For this review, take the finished solid that the model builds, in its own axes (mm). A direction names the side the tool comes from. Round coordinates to 2 decimals unless told otherwise and drop trailing zeros. Write each loop counter-clockwise with the first axis right and the second up, starting at its lowest first coordinate (ties: lowest second). Pieces come first, ordered by that corner, then holes. Notation, with made-up numbers: M -40,64 L 3,64 A38 ccw 3,102 Z; hole C -9,9 d10. An arc over 180 degrees is marked long. Use one line per item in the form item = value. Start each with the question number.
Item 1: For P1, Ø1.5, axis at x = -26.5, y = 5, coming from the -Z side; P2, Ø1.5, axis at x = -28.5, z = 15, coming from the +Y side; P3, Ø3, axis at x = -38.5, y = 2.5, coming from the +Z side; P4, Ø6, axis at y = 3.5, z = 13.5, coming from the +X side, all flat-tipped, find the tip position at first contact; note any pin that passes through.
Item 2: Add section C-C (x = -50.5). State the section outline as (y, z) points (3 decimals), and give its area (3 significant figures).
Item 3: For faces 4 (the flat face through (-48, 0, -3)), 5 (the flat face through (-63.5, -1, 10)), 6 (the flat face through (-32, -6.35, 13)), 7 (the flat face through (-32, 3, 6.35)), 8 (the flat face through (-31.75, 5, -2)), list the 3-axis set-ups (+Z, -Z, +X, -X, +Y, -Y) from which the entire face can be reached by the end or side of a thin tool; tool diameter is ignored.
Item 4: Draft analysis for pull direction Z (two halves, no side actions). For faces 1 (the flat face through (-32, 0, 16)), 2 (the cylindrical face through (-47.847, 2.296, -4.865)), 3 (the flat face through (-48, 3, -6.35)), state which applies: released by +Z, released by -Z, zero draft, split by the parting line, or undercut.
Item 5: For line 1 (Z direction, x = -24, y = 0.75); line 2 (Z direction, x = -60.5, y = -2.5); line 3 (Y direction, x = -9.5, z = 14.5), list the stretches that pass through material, from the lowest coordinate up. Write a range as [from, to].
Item 6: Add section D-D (z = 8). State the section outline as (x, y) points.
Item 7: Add section A-A (y = 4.5). State the section outline as (x, z) points.
Item 8: Add section B-B (x = -31). State the section outline as (y, z) points, and give its area (3 significant figures).
from build123d import *

# Parameters (mm, degrees)
F0_W     = 63.5
F0_H     = 25.4
F1_DEPTH = 6.35
F2_W     = 63.5
F2_H     = 6.35
F3_DEPTH = 6.35
F4_W     = 63.5
F4_H     = 6.35
F5_DEPTH = 6.35
F6_R     = 1.905
F7_DEPTH = 63.501
F8_W     = 31.75
F8_H     = 6.35
F9_DEPTH = 25.4


with BuildPart() as f1:
    # F0 (on Front) → F1 (new body)
    with BuildSketch(Plane.XZ):
        with Locations((-31.75, 12.7)):
            Rectangle(F0_W, F0_H)
    extrude(amount=F1_DEPTH)

    # F2 (on Front) → F3 (join)
    with BuildSketch(Plane.XZ):
        with Locations((-31.75, 3.175)):
            Rectangle(F2_W, F2_H)
    extrude(amount=-F3_DEPTH)

    # F4 (on face) → F5 (join)
    with BuildSketch(Plane(origin=(0, 0, 0), x_dir=(1, 0, 0), z_dir=(0, 0, -1))):
        with Locations((-31.75, -3.175)):
            Rectangle(F4_W, F4_H)
    extrude(amount=F5_DEPTH)

    # F6 (on face) → F7 (cut, through all)
    with BuildSketch(Plane(origin=(-63.5, 0, 0), x_dir=(0, -1, 0), z_dir=(-1, 0, 0))):
        with Locations((-3.175, -3.175)):
            Circle(F6_R)
    extrude(amount=-F7_DEPTH, mode=Mode.SUBTRACT)

    # F8 (on face) → F9 (cut)
    with BuildSketch(Plane.XZ):
        with Locations((-15.875, -3.175)):
            Rectangle(F8_W, F8_H)
    extrude(amount=-F9_DEPTH, mode=Mode.SUBTRACT)


solid = f1.part
Calculated:
q1.P1 = 0
q1.P2 = 0
q1.P3 = 6.35
q1.P4 = through
q2.outline = M -6.35,0 L 0,0 L 0,-6.35 L 6.35,-6.35 L 6.35,6.35 L 0,6.35 L 0,25.4 L -6.35,25.4 Z; hole C 3.175,-3.175 d3.81
q2.area = 231 mm^2
q3.face_4 = -Z, +X, -X, -Y
q3.face_5 = +Z, -Z, -X, +Y, -Y
q3.face_6 = +Z, -Z, +X, -X, -Y
q3.face_7 = +Z, +X, -X, +Y
q3.face_8 = -Z, +X, +Y, -Y
q4.face_1 = zero draft
q4.face_2 = undercut
q4.face_3 = released by -Z
q5.line_1 = [0, 6.35]
q5.line_2 = [0, 25.4]
q5.line_3 = [-6.35, 0]
q6.outline = M -63.5,-6.35 L 0,-6.35 L 0,0 L -63.5,0 Z
q7.outline = M -63.5,-6.35 L -31.75,-6.35 L -31.75,-4.54 L -63.5,-4.54 Z; M -63.5,-1.81 L -31.75,-1.81 L -31.75,0 L 0,0 L 0,6.35 L -63.5,6.35 Z
q8.outline = M -6.35,0 L 6.35,0 L 6.35,6.35 L 0,6.35 L 0,25.4 L -6.35,25.4 Z
q8.area = 202 mm^2
